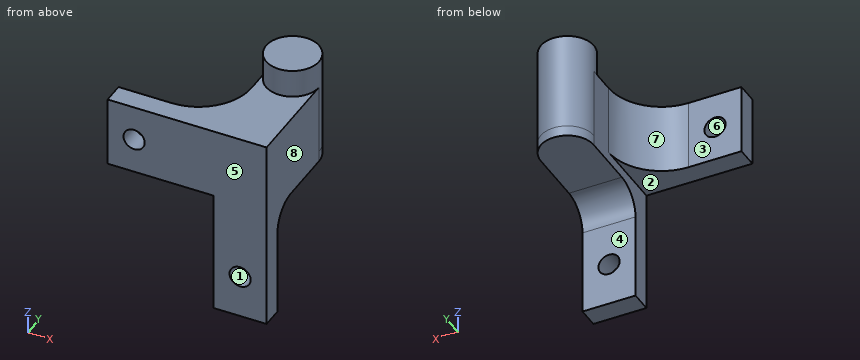
from build123d import *

# Parameters (mm, degrees)
BOSS_EXTRUDE1_DEPTH = 20
SKETCH3_R           = 7.5
BOSS_EXTRUDE3_DEPTH = 8
BOSS_EXTRUDE4_DEPTH = 15
BOSS_EXTRUDE5_START = 3
SKETCH5_R           = 7.5
BOSS_EXTRUDE5_DEPTH = 3
SKETCH6_R           = 3
CUT_EXTRUDE1_DEPTH  = 60.678304265


with BuildPart() as part:
    # Sketch1 → Boss-Extrude1 (new body)
    with BuildSketch(Plane.XY):
        with BuildLine():
            Line((-7.5, 0), (-7.5, -8))
            ThreePointArc((-7.5, -8), (-11.893398282, -18.606601718), (-22.5, -23))
            Line((-22.5, -23), (-37.5, -23))
            Line((-37.5, -23), (-37.5, -29))
            Line((-37.5, -29), (7.5, -29))
            Line((7.5, -29), (7.5, -23))
            Line((7.5, -23), (7.5, -8))
            Line((7.5, -8), (7.5, 0))
            ThreePointArc((7.5, 0), (0, 7.5), (-7.5, 0))
        make_face()
    extrude(amount=BOSS_EXTRUDE1_DEPTH)

    # Sketch3 → Boss-Extrude3 (add)
    with BuildSketch(Plane.XY.offset(20)):
        Circle(SKETCH3_R)
    extrude(amount=BOSS_EXTRUDE3_DEPTH)

    # Sketch4 → Boss-Extrude4 (add)
    with BuildSketch(Plane(origin=(7.5, 0, 0), x_dir=(0, 0, -1), z_dir=(1, 0, 0))):
        with BuildLine():
            Line((0, -29), (35, -29))
            Line((35, -29), (35, -23))
            Line((35, -23), (10.5, -23))
            ThreePointArc((10.5, -23), (5.196699141, -20.803300859), (3, -15.5))
            Line((3, -15.5), (3, 0))
            Line((3, 0), (0, 0))
            Line((0, 0), (0, -29))
        make_face()
    extrude(amount=-BOSS_EXTRUDE4_DEPTH)

    # Sketch5 → Boss-Extrude5 (add)
    with BuildSketch(Plane(origin=(0, 0, 0), x_dir=(-1, 0, 0), z_dir=(0, 0, -1)).offset(BOSS_EXTRUDE5_START)):
        with Locations(Location((0, 0, 0), (0, 0, 180))):
            Circle(SKETCH5_R)
    extrude(amount=-BOSS_EXTRUDE5_DEPTH)

    # Sketch6 → Cut-Extrude1 (cut, through all)
    with BuildSketch(Plane(origin=(0, -23, 0), x_dir=(1, 0, 0), z_dir=(0, 1, 0))):
        with Locations(Location((0, 22.783810394, 0), (0, 0, 270))):
            Circle(SKETCH6_R)
        with Locations(Location((-30, -10, 0), (0, 0, 270))):
            Circle(SKETCH6_R)
    extrude(amount=-CUT_EXTRUDE1_DEPTH, mode=Mode.SUBTRACT)


solid = part.part
Model file for the job. Use its own axes, mm. Face numbers are marked on the shaded views. A direction names the side the tool comes from. Give positions to 0.01 mm unless a question says otherwise; leave off trailing zeros. Loops run counter-clockwise (first coordinate to the right, second up) from the corner with the lowest first, then second, coordinate; pieces in that order, holes last.
1) Saw through at C-C (y = -1). Write the cut outline in (x, z), plus the area to 3 significant figures.
2) Saw through at B-B (z = 10). Write the cut outline in (x, y).
3) Tool access for the marked faces 1, 2, 3 and 4: list every direction of +Z, -Z, +X, -X, +Y, -Y with a clear straight run to the whole face (end or side of a thin tool).
4) Wall check: line 1 (Z direction, x = 1, y = 5); line 2 (X direction, y = -3, z = -2); line 3 (X direction, y = -27, z = -23.5). Give the ranges that are in metal, low to high.
5) Pull direction X, two halves, no side cores. Call the marked faces 5, 6, 7 and 8: +X half, -X half, draft (parallel to the pull), parting line (faces both ways), or undercut.
6) Saw through at D-D (z = 19). Write the cut outline in (x, y), plus the area to 3 significant figures.
7) Flat gauge pins, fed straight in: pin 1 Ø8 at (x, z) = (0, -22.78) entering from +Y; pin 2 Ø3 at (y, z) = (3.5, 10.5) entering from -X; pin 3 Ø10.5 at (x, y) = (-23.5, -16) entering from -Z; pin 4 Ø8 at (x, z) = (-18, 16) entering from +Y. Where does each tip first touch, or does it go through?
8) Saw through at A-A (x = 0). Write the cut outline in (y, z), plus the area to 3 significant figures.
Answer block:
1. outline: (-7.5, -3) - (7.5, -3) - (7.5, 20) - (7.43, 20) - (7.43, 28) - (-7.43, 28) - (-7.43, 20) - (-7.5, 20) - close
1. area: 464 mm2
2. outline: (-37.5, -29) - (-33, -29) - (-33, -23) - (-37.5, -23) - close; (-27, -29) - (7.5, -29) - (7.5, 0) arc R7.5 ccw to (-7.5, 0) - (-7.5, -8) arc R15 cw to (-22.5, -23) - (-27, -23) - close
3. face 1: +Y, -Y
3. face 2: -Z, -X, +Y, -Y
3. face 3: +Z, -Z, -X, +Y
3. face 4: -Z, +X, -X, +Y
4. line 1: z = -3 to 28
4. line 2: x = -7.5 to 7.5
4. line 3: x = -7.5 to -2.91, 2.91 to 7.5
5. face 5: draft
5. face 6: undercut
5. face 7: -X half
5. face 8: +X half
6. outline: (-37.5, -29) - (7.5, -29) - (7.5, 0) arc R7.5 ccw to (-7.5, 0) - (-7.5, -8) arc R15 cw to (-22.5, -23) - (-37.5, -23) - close
6. area: 752 mm2
7. pin 1: stops at y = -23
7. pin 2: stops at x = -7.23
7. pin 3: passes through
7. pin 4: stops at y = -20.36
8. outline: (-29, -35) - (-23, -35) - (-23, -25.78) - (-29, -25.78) - close; (-29, -19.78) - (-23, -19.78) - (-23, -10.5) arc R7.5 cw to (-15.5, -3) - (7.5, -3) - (7.5, 28) - (-7.5, 28) - (-7.5, 20) - (-29, 20) - close
8. area: 1,130 mm2
